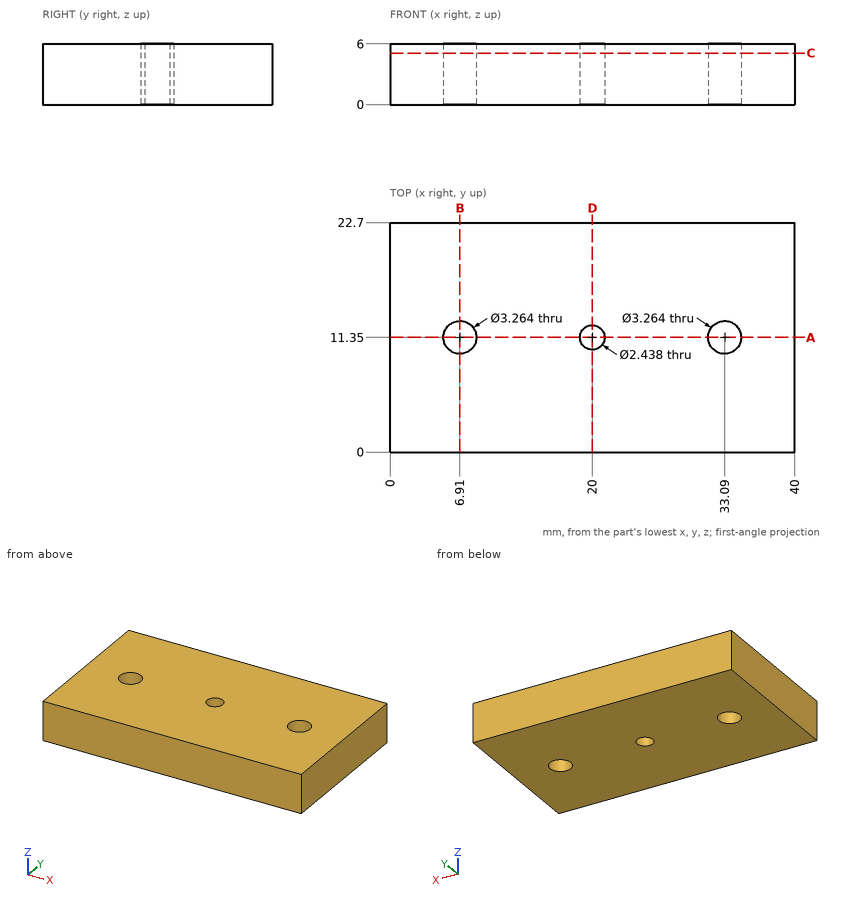
Print and shaded views of the part. All mm, measured from the part's lowest x, y and z. Give positions to 0.01 mm unless a question says otherwise; leave off trailing zeros. Loops run counter-clockwise (first coordinate to the right, second up) from the corner with the lowest first, then second, coordinate; pieces in that order, holes last. Notation, with made-up numbers: (-4, -11.5) - (3, -11.5) arc R29 ccw to (3, 16.5) - close; hole circle Ø6 at (65.25, 84.5). An arc over 180 degrees is marked (long way). One line per item, written item: value. Start each with the question number.
1. Slice it at D-D (x = 20). List the corners of the cut face in (y, z).
2. Slice it at B-B (x = 6.91). List the corners of the cut face in (y, z).
3. Probe L1, parallel to X at y = 11.5, z = 4.85 (1 decimal); L2, parallel to Y at x = 6.91, z = 4.3; L3, parallel to Y at x = 20, z = 4.4. List the from-to ranges inside material, lowest first. Write a range as from..to.
4. Slice it at A-A (y = 11.35). List the corners of the cut face in (x, z).
5. Pin check, flat tip, straight feed: pin 1 (2.5 mm diameter, centred on x = 33.09, y = 11.35, fed in from -Z). Stop position of the tip, or through.
6. Slice it at C-C (z = 5.1). List the corners of the cut face in (x, y).
Solution:
1. outline: (0, 0) - (10.13, 0) - (10.13, 6) - (0, 6) - close; (12.57, 0) - (22.7, 0) - (22.7, 6) - (12.57, 6) - close
2. outline: (0, 0) - (9.72, 0) - (9.72, 6) - (0, 6) - close; (12.98, 0) - (22.7, 0) - (22.7, 6) - (12.98, 6) - close
3. L1: x = 0..5.3, 8.5..18.8, 21.2..31.5, 34.7..40
3. L2: y = 0..9.72, 12.98..22.7
3. L3: y = 0..10.13, 12.57..22.7
4. outline: (0, 0) - (5.28, 0) - (5.28, 6) - (0, 6) - close; (8.54, 0) - (18.78, 0) - (18.78, 6) - (8.54, 6) - close; (21.22, 0) - (31.46, 0) - (31.46, 6) - (21.22, 6) - close; (34.72, 0) - (40, 0) - (40, 6) - (34.72, 6) - close
5. pin 1: passes through
6. outline: (0, 0) - (40, 0) - (40, 22.7) - (0, 22.7) - close; hole circle Ø3.26 at (6.91, 11.35); hole circle Ø2.44 at (20, 11.35); hole circle Ø3.26 at (33.09, 11.35)
